Model file for the job. Use its own axes, mm. A direction names the side the tool comes from. Round coordinates to 2 decimals unless told otherwise and drop trailing zeros. Loops run counter-clockwise (first coordinate to the right, second up) from the corner with the lowest first, then second, coordinate; pieces in that order, holes last. Notation, with made-up numbers: (-8.5, 71.25) - (24.5, 71.25) arc R31 cw to (24.5, 101.25) - close; hole circle Ø6 at (7.5, 48.5). An arc over 180 degrees is marked (long way). Use one line per item in the form item = value.
from build123d import *

# Parameters (mm, degrees)
F1_DEPTH = 7
F3_DEPTH = 3.6
F4_START = 1.5
F4_DEPTH = 2.1


with BuildPart() as f1:
    # F0 (on Front) → F1 (new body, symmetric)
    with BuildSketch(Plane.XZ):
        Polygon((-75, 0), (0, 0), (0, 6.4), (-2.7, 6.4), (-2.7, 2.5), (-5.7, 2.5), (-5.7, 5.1), (-4.5, 5.1), (-4.5, 6.4), (-4.5, 7.1), (-7.1, 6.4), (-19.2, 6.4), (-19.2, 6.9), (-31.7, 6.9), (-31.2, 6.4), (-28.7, 3.9), (-47.2, 3.9), (-44.7, 6.4), (-44.2, 6.9), (-56.7, 6.9), (-56.7, 6.4), (-68.1, 6.4), (-70.7, 7.1), (-70.7, 6.4), (-70.7, 5.1), (-69.5, 5.1), (-69.5, 2.5), (-72.5, 2.5), (-72.5, 6.4), (-75, 6.4), align=None)
    extrude(amount=F1_DEPTH, both=True)

    # F2 (on face) → F3 (join)
    with BuildSketch(Plane(origin=(0, 0, 0), x_dir=(1, 0, 0), z_dir=(0, 0, -1))):
        with BuildLine():
            ThreePointArc((-34.5395570389, -0.4855692269), (-34.5099056133, -0.2435889127), (-34.5, 0))
            ThreePointArc((-34.5, 0), (-34.5099056133, 0.2435889127), (-34.5395570389, 0.4855692269))
            ThreePointArc((-34.5395570389, 0.4855692269), (-35.3786796564, 2.1213203436), (-37.0144307731, 2.9604429611))
            ThreePointArc((-37.0144307731, 2.9604429611), (-37.5, 3), (-37.9855692269, 2.9604429611))
            ThreePointArc((-37.9855692269, 2.9604429611), (-39.6213203436, 2.1213203436), (-40.4604429611, 0.4855692269))
            ThreePointArc((-40.4604429611, 0.4855692269), (-40.5, 0), (-40.4604429611, -0.4855692269))
            ThreePointArc((-40.4604429611, -0.4855692269), (-39.6213203436, -2.1213203436), (-37.9855692269, -2.9604429611))
            ThreePointArc((-37.9855692269, -2.9604429611), (-37.5, -3), (-37.0144307731, -2.9604429611))
            ThreePointArc((-37.0144307731, -2.9604429611), (-35.3786796564, -2.1213203436), (-34.5395570389, -0.4855692269))
        make_face()
    extrude(amount=F3_DEPTH)

    # F2 (on face) → F4 (join)
    with BuildSketch(Plane(origin=(0, 0, 0), x_dir=(1, 0, 0), z_dir=(0, 0, -1)).offset(F4_START)):
        with BuildLine():
            ThreePointArc((-40.4604429611, 0.4855692269), (-39.6213203436, 2.1213203436), (-37.9855692269, 2.9604429611))
            Line((-37.9855692269, 2.9604429611), (-41.9634402584, 6.9383139926))
            ThreePointArc((-41.9634402584, 6.9383139926), (-43.3336309448, 5.8336309448), (-44.4383139926, 4.4634402584))
            Line((-44.4383139926, 4.4634402584), (-40.4604429611, 0.4855692269))
        make_face()
        with BuildLine():
            ThreePointArc((-37.0144307731, 2.9604429611), (-35.3786796564, 2.1213203436), (-34.5395570389, 0.4855692269))
            Line((-34.5395570389, 0.4855692269), (-30.5616860074, 4.4634402584))
            ThreePointArc((-30.5616860074, 4.4634402584), (-31.6663690552, 5.8336309448), (-33.0365597416, 6.9383139926))
            Line((-33.0365597416, 6.9383139926), (-37.0144307731, 2.9604429611))
        make_face()
        with BuildLine():
            Line((-41.9634402584, -6.9383139926), (-37.9855692269, -2.9604429611))
            ThreePointArc((-37.9855692269, -2.9604429611), (-39.6213203436, -2.1213203436), (-40.4604429611, -0.4855692269))
            Line((-40.4604429611, -0.4855692269), (-44.4383139926, -4.4634402584))
            ThreePointArc((-44.4383139926, -4.4634402584), (-43.3336309448, -5.8336309448), (-41.9634402584, -6.9383139926))
        make_face()
        with BuildLine():
            Line((-30.5616860074, -4.4634402584), (-34.5395570389, -0.4855692269))
            ThreePointArc((-34.5395570389, -0.4855692269), (-35.3786796564, -2.1213203436), (-37.0144307731, -2.9604429611))
            Line((-37.0144307731, -2.9604429611), (-33.0365597416, -6.9383139926))
            ThreePointArc((-33.0365597416, -6.9383139926), (-31.6663690552, -5.8336309448), (-30.5616860074, -4.4634402584))
        make_face()
    extrude(amount=F4_DEPTH)


solid = f1.part
1. Cut at C-C, the plane x = -13. Give the cut face in (y, z).
Geometry check:
outline = (-7, 0) - (7, 0) - (7, 6.4) - (-7, 6.4) - close
2. Flat gauge pins, fed straight in: pin 1 (2.5 mm diameter, centred on x = -70.5, y = 2.5, fed in from +Z); pin 2 (2 mm diameter, centred on x = -1.5, y = 3.5, fed in from +Z); pin 3 (4 mm diameter, centred on x = -41, y = -1, fed in from +Z). Where does each tip first touch, or does it go through?
Geometry check:
pin_1 = 7.1
pin_2 = 6.4
pin_3 = 3.9
3. Tool access for faces 1 (the flat face through (-34, -4, -1.5)), 2 (the flat face through (-5.782, -0.098, 6.755)), 3 (the flat face through (-39.947, -4.922, -2.535)), 4 (the cylindrical face through (-31.65, -5.82, -2.54)), 5 (the flat face through (-34, 4, -1.5)): list every direction of +Z, -Z, +X, -X, +Y, -Y with a clear straight run to the whole face (end or side of a thin tool).
Geometry check:
face_1 = +X, -Y
face_2 = +Z, +Y, -Y
face_3 = -Z, -Y
face_4 = -Z, +X, -Y
face_5 = +X, +Y
4. Cut at D-D, the plane x = -28. Give the cut face in (y, z).
Geometry check:
outline = (-7, 0) - (7, 0) - (7, 6.9) - (-7, 6.9) - close
5. Wall check: probe 1 along X at (y, z) = (-0.5, 3.75); probe 2 along X at (y, z) = (1, 5.25); probe 3 along Z at (x, y) = (-58.5, -2). Give the ranges that are in metal, low to high.
Geometry check:
probe_1 = -75 to -72.5, -69.5 to -5.7, -2.7 to 0
probe_2 = -75 to -72.5, -70.7 to -45.85, -30.05 to -4.5, -2.7 to 0
probe_3 = 0 to 6.4
6. Cut at A-A, the plane z = -0.75. Give the cut face in (x, y).
Geometry check:
outline = circle Ø6 at (-37.5, 0)
7. Pull direction Z, two halves, no side cores. Call faces 6 (the flat face through (-70, 0, 5.1)), 7 (the flat face through (-38, 7, 3.6)), 8 (the flat face through (-25, 0, 6.9)): +Z half, -Z half, draft (parallel to the pull), parting line (faces both ways), or undercut.
Geometry check:
face_6 = undercut
face_7 = draft
face_8 = +Z half
